Verification items for this drawing (mm, ordinates from the low corner). A direction names the side the tool comes from. Round coordinates to 2 decimals unless told otherwise and drop trailing zeros. Order: outer loops, then holes, each group sorted by start corner. A loop starts at its lowest first (then second) coordinate and runs counter-clockwise, first axis right, second up. Notation, with made-up numbers: M 21,-26.75 L 39,-26.75 A16 ccw 39,-5.75 Z; hole C -10,42 d4. An arc over 180 degrees is marked long. One line per item, written item: value. Start each with the question number.
(1) Cross-section at C-C, the plane z = 2.25. Enter the section's corners in (x, y).
(2) Cross-section at A-A, the plane y = 16. Enter the section's corners in (x, z), and give its area (4 significant figures).
(3) Access from +Z, -Z, +X, -X, +Y, -Y to the whole of each face (thin tool, end or side, straight path). Record for the marked faces 4 and 5.
(4) Thickness scan on L1, parallel to Y at x = 10, z = 13.75; L2, parallel to Y at x = 8, z = 8; L3, parallel to Z at x = 10.5, y = 100. Record the ranges inside material, lowest first.
(5) Release check for a two-part mould opening along Y. For the marked faces 1, 2 and 3 record: released by +Y, released by -Y, zero draft, split by the parting line, or undercut.
(6) Cross-section at B-B, the plane x = 10. Enter the section's corners in (y, z).
(7) Depth check by flat-ended pin: pin 1 Ø9 at (x, y) = (10, 16) entering from +Z; pin 2 Ø12 at (x, y) = (14, 100.5) entering from -Z. Enter the tip coordinate at first touch or a pass-through.
(8) Cross-section at D-D, the plane x = 16.5. Enter the section's corners in (y, z).
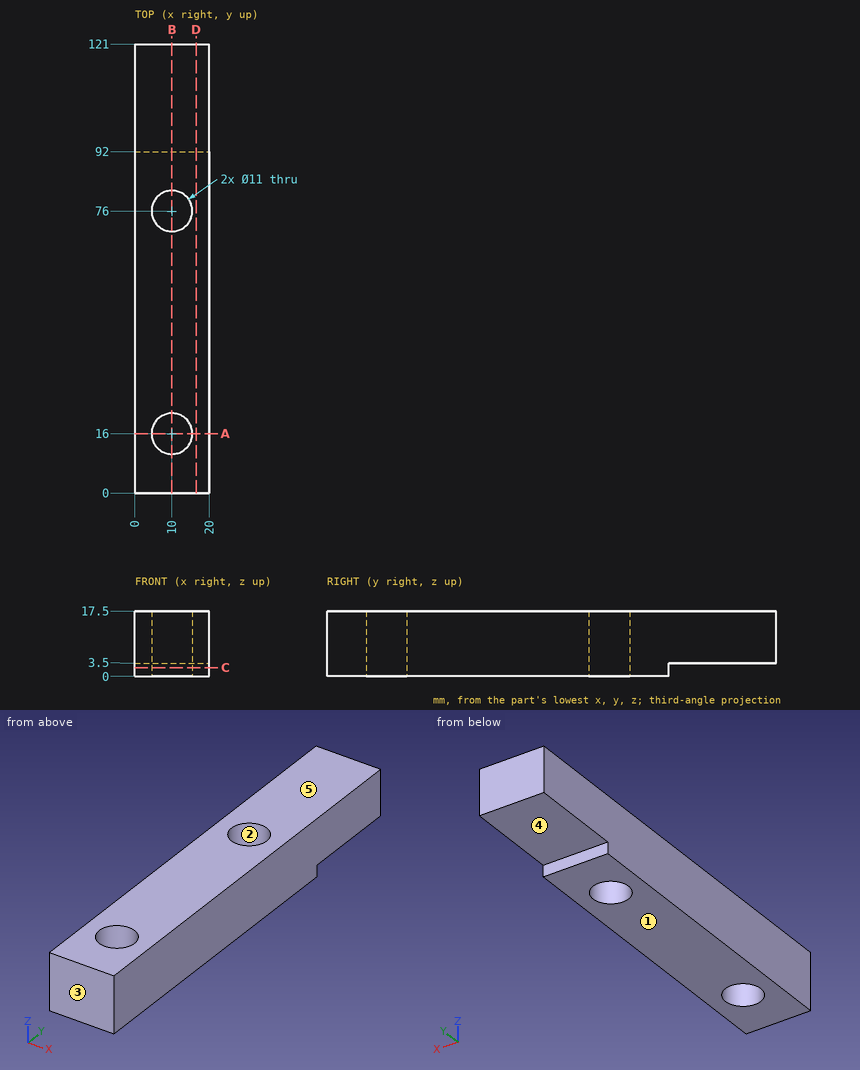
Values found:
1. outline: M 0,0 L 20,0 L 20,92 L 0,92 Z; hole C 10,16 d11; hole C 10,76 d11
2. outline: M 0,0 L 4.5,0 L 4.5,17.5 L 0,17.5 Z; M 15.5,0 L 20,0 L 20,17.5 L 15.5,17.5 Z
2. area: 157.5 mm^2
3. face 4: -Z, +X, -X, +Y
3. face 5: +Z, +X, -X, +Y, -Y
4. L1: 0 to 10.5, 21.5 to 70.5, 81.5 to 121
4. L2: 0 to 10.88, 21.12 to 70.88, 81.12 to 121
4. L3: 3.5 to 17.5
5. face 1: zero draft
5. face 2: undercut
5. face 3: released by -Y
6. outline: M 0,0 L 10.5,0 L 10.5,17.5 L 0,17.5 Z; M 21.5,0 L 70.5,0 L 70.5,17.5 L 21.5,17.5 Z; M 81.5,0 L 92,0 L 92,3.5 L 121,3.5 L 121,17.5 L 81.5,17.5 Z
7. pin 1: through
7. pin 2: z = 3.5
8. outline: M 0,0 L 92,0 L 92,3.5 L 121,3.5 L 121,17.5 L 0,17.5 Z
